For this review, take the finished solid that the model builds, in its own axes (mm). Round coordinates to 2 decimals unless told otherwise and drop trailing zeros. Write each loop counter-clockwise with the first axis right and the second up, starting at its lowest first coordinate (ties: lowest second). Pieces come first, ordered by that corner, then holes. Notation, with made-up numbers: (-16, 84) -> (-3, 84) arc R28 ccw to (-3, 105) -> close; hole circle Ø4 at (32.25, -13.5). An arc over 180 degrees is marked (long way). Answer in a Markdown table with one row per item. Add a question column.
```python
from build123d import *

# Parameters (mm, degrees)
F0_R     = 10.9982
F1_DEPTH = 6.35


with BuildPart() as f1:
    # F0 (on Front) → F1 (new body)
    with BuildSketch(Plane.XZ):
        with BuildLine():
            ThreePointArc((-7.1437498937, -12.3733380179), (7.1437500531, -12.3733379259), (14.2875, 0))
            ThreePointArc((14.2875, 0), (7.1437499995, 12.3733379569), (-7.143750001, 12.373337956))
            ThreePointArc((-7.143750001, 12.373337956), (-14.2875, -6.19e-08), (-7.1437498937, -12.3733380179))
        make_face()
        Circle(F0_R, mode=Mode.SUBTRACT)
        with BuildLine():
            ThreePointArc((23.01875, -15.1229686136), (16.6270313864, -8.73125), (14.2875, 0))
            ThreePointArc((14.2875, 0), (7.1437500531, -12.3733379259), (-7.1437498937, -12.3733380179))
            ThreePointArc((-7.1437498937, -12.3733380179), (-0.7520313557, -18.7650566233), (1.5875, -27.4963065702))
            ThreePointArc((1.5875, -27.4963065702), (8.73125, -15.1229686136), (23.01875, -15.1229686136))
        make_face()
        with BuildLine():
            ThreePointArc((-7.143750001, 12.373337956), (7.1437499995, 12.3733379569), (14.2875, 0))
            ThreePointArc((14.2875, 0), (16.6270313864, 8.73125), (23.01875, 15.1229686136))
            ThreePointArc((23.01875, 15.1229686136), (8.73125, 15.1229686136), (1.5875, 27.4963065702))
            ThreePointArc((1.5875, 27.4963065702), (-0.7520313867, 18.7650565696), (-7.143750001, 12.373337956))
        make_face()
        with BuildLine():
            ThreePointArc((-7.1437498937, -12.3733380179), (-14.2875, -6.19e-08), (-7.143750001, 12.373337956))
            ThreePointArc((-7.143750001, 12.373337956), (-15.8750000006, 10.0338065702), (-24.60625, 12.3733379566))
            ThreePointArc((-24.60625, 12.3733379566), (-19.3766620434, 7.14375), (-17.4625, 0))
            ThreePointArc((-17.4625, 0), (-19.3766620434, -7.14375), (-24.60625, -12.3733379566))
            ThreePointArc((-24.60625, -12.3733379566), (-15.8749999387, -10.0338065702), (-7.1437498937, -12.3733380179))
        make_face()
        with BuildLine():
            ThreePointArc((1.5875, 27.4963065702), (8.73125, 15.1229686136), (23.01875, 15.1229686136))
            ThreePointArc((23.01875, 15.1229686136), (28.2483379566, 20.3525565702), (30.1625, 27.4963065702))
            ThreePointArc((30.1625, 27.4963065702), (15.875, 41.7838065702), (1.5875, 27.4963065702))
        make_face()
        with Locations((15.875, 27.4963065702)):
            Circle(F0_R, mode=Mode.SUBTRACT)
        with BuildLine():
            ThreePointArc((30.1625, -27.4963065702), (28.2483379566, -20.3525565702), (23.01875, -15.1229686136))
            ThreePointArc((23.01875, -15.1229686136), (8.73125, -15.1229686136), (1.5875, -27.4963065702))
            ThreePointArc((1.5875, -27.4963065702), (15.875, -41.7838065702), (30.1625, -27.4963065702))
        make_face()
        with Locations((15.875, -27.4963065702)):
            Circle(F0_R, mode=Mode.SUBTRACT)
        with BuildLine():
            ThreePointArc((-17.4625, 0), (-19.3766620434, 7.14375), (-24.60625, 12.3733379566))
            ThreePointArc((-24.60625, 12.3733379566), (-46.0375, 0), (-24.60625, -12.3733379566))
            ThreePointArc((-24.60625, -12.3733379566), (-19.3766620434, -7.14375), (-17.4625, 0))
        make_face()
        with Locations((-31.75, 0)):
            Circle(F0_R, mode=Mode.SUBTRACT)
    extrude(amount=F1_DEPTH)


solid = f1.part
```
1. We need section B-B (y = -2). Count the separate pieces of the cut face and the enclosed holes in it, plus the area to 3 significant figures.
2. The part is to be moulded in two halves that separate along Z. For faces 1 (the flat face through (-11, 0, -3)), 2 (the cylindrical face through (7, -3, 21)), 3 (the cylindrical face through (-6.923, -3.131, 12.503)), 4 (the cylindrical face through (-42.738, -3.131, 0.484)), say which applies: pulls with the +Z half, pulls with the -Z half, needs draft (parallel to the pull), parting line crosses it, or undercut.
3. For L1, parallel to X at y = -0.5, z = 0.5; L2, parallel to Z at x = 19.5, y = -5.75; L3, parallel to Z at x = 13.5, y = -3, list the stretches that pass through material, from the lowest coordinate up. Write a range as [from, to].
4. We need section A-A (x = -31.75). Write out the cut boundary in (y, z), plus the area to 3 significant figures.
5. Clearance check with flat-ended pins moving along their axes: pin 1 Ø1.5 at (x, y) = (17.5, -4) entering from -Z; pin 2 Ø2 at (x, y) = (-35, -1) entering from +Z; pin 3 Ø3 at (x, y) = (-35, -1) entering from -Z; pin 4 Ø20 at (x, z) = (0, 0) entering from +Y. State where each tip first meets the part, or that it passes through.
Response:
| question | item | result |
|---|---|---|
| 1 | separate pieces | 1 |
| 1 | enclosed holes | 4 |
| 1 | area | 1,420 mm2 |
| 2 | face 1 | needs draft |
| 2 | face 2 | undercut |
| 2 | face 3 | pulls with the +Z half |
| 2 | face 4 | undercut |
| 3 | L1 | [-46.03, -42.74], [-20.76, -10.99], [10.99, 14.29] |
| 3 | L2 | [-41.32, -37.88], [-17.11, -12.44], [12.44, 17.11], [37.88, 41.32] |
| 3 | L3 | [-41.59, -38.24], [-16.76, 16.76], [38.24, 41.59] |
| 4 | outline | (-6.35, -14.29) -> (0, -14.29) -> (0, -11) -> (-6.35, -11) -> close; (-6.35, 11) -> (0, 11) -> (0, 14.29) -> (-6.35, 14.29) -> close |
| 4 | area | 41.8 mm2 |
| 5 | pin 1 | z = -41.76 |
| 5 | pin 2 | z = 14.11 |
| 5 | pin 3 | z = -14.18 |
| 5 | pin 4 | through |
